Work out the finished part from the listing and answer in its coordinate system (mm). Coordinates: 2 decimals unless noted, no trailing zeros. Loops run counter-clockwise (first coordinate to the right, second up) from the corner with the lowest first, then second, coordinate; pieces in that order, holes last. Notation, with made-up numbers: (56.25, -29.5) -> (80.25, -29.5) arc R25 cw to (80.25, -17.5) -> close; hole circle Ø11 at (73, 47.25). An arc over 180 degrees is marked (long way). Use a Markdown table: item, result.
from build123d import *

# Parameters (mm, degrees)
F0_R     = 12.6233535656
F0_R_2   = 19.05
F1_DEPTH = 3.175


with BuildPart() as f1:
    # F0 (on Front) → F1 (new body)
    with BuildSketch(Plane.XZ):
        with BuildLine():
            ThreePointArc((68.11386007, -24.7914176064), (71.3840419736, -12.586932592), (72.485255884, 0))
            ThreePointArc((72.485255884, 0), (71.3840419736, 12.586932592), (68.11386007, 24.7914176064))
            ThreePointArc((68.11386007, 24.7914176064), (62.7740729954, 36.242627942), (55.526927478, 46.5926243672))
            ThreePointArc((55.526927478, 46.5926243672), (46.5926243672, 55.526927478), (36.242627942, 62.7740729954))
            ThreePointArc((36.242627942, 62.7740729954), (24.7914176064, 68.11386007), (12.586932592, 71.3840419736))
            ThreePointArc((12.586932592, 71.3840419736), (0, 72.485255884), (-12.586932592, 71.3840419736))
            ThreePointArc((-12.586932592, 71.3840419736), (-24.7914176064, 68.11386007), (-36.242627942, 62.7740729954))
            ThreePointArc((-36.242627942, 62.7740729954), (-46.5926243672, 55.526927478), (-55.526927478, 46.5926243672))
            ThreePointArc((-55.526927478, 46.5926243672), (-62.7740729954, 36.242627942), (-68.11386007, 24.7914176064))
            ThreePointArc((-68.11386007, 24.7914176064), (-71.3840419736, 12.586932592), (-72.485255884, 0))
            ThreePointArc((-72.485255884, 0), (-71.3840419736, -12.586932592), (-68.11386007, -24.7914176064))
            ThreePointArc((-68.11386007, -24.7914176064), (-62.7740729954, -36.242627942), (-55.526927478, -46.5926243672))
            ThreePointArc((-55.526927478, -46.5926243672), (-46.5926243672, -55.526927478), (-36.242627942, -62.7740729954))
            ThreePointArc((-36.242627942, -62.7740729954), (-24.7914176064, -68.11386007), (-12.586932592, -71.3840419736))
            ThreePointArc((-12.586932592, -71.3840419736), (0, -72.485255884), (12.586932592, -71.3840419736))
            ThreePointArc((12.586932592, -71.3840419736), (24.7914176064, -68.11386007), (36.242627942, -62.7740729954))
            ThreePointArc((36.242627942, -62.7740729954), (46.5926243672, -55.526927478), (55.526927478, -46.5926243672))
            ThreePointArc((55.526927478, -46.5926243672), (62.7740729954, -36.242627942), (68.11386007, -24.7914176064))
        make_face()
        with Locations((-25.4, -38.1)):
            Circle(F0_R, mode=Mode.SUBTRACT)
        with Locations((25.4, -38.1)):
            Circle(F0_R, mode=Mode.SUBTRACT)
        with Locations((-25.4, 38.1)):
            Circle(F0_R, mode=Mode.SUBTRACT)
        Circle(F0_R_2, mode=Mode.SUBTRACT)
        with Locations((25.4, 38.1)):
            Circle(F0_R, mode=Mode.SUBTRACT)
        with BuildLine():
            Line((87.4346938634, -13.8457773117), (72.485255884, 0))
            ThreePointArc((72.485255884, 0), (71.3840419736, -12.586932592), (68.11386007, -24.7914176064))
            Line((68.11386007, -24.7914176064), (87.4346938634, -13.8457773117))
        make_face()
        with BuildLine():
            ThreePointArc((68.11386007, 24.7914176064), (71.3840419736, 12.586932592), (72.485255884, 0))
            Line((72.485255884, 0), (86.8972713647, 16.893651758))
            Line((86.8972713647, 16.893651758), (68.11386007, 24.7914176064))
        make_face()
        with BuildLine():
            ThreePointArc((55.526927478, 46.5926243672), (62.7740729954, 36.242627942), (68.11386007, 24.7914176064))
            Line((68.11386007, 24.7914176064), (75.8787554723, 45.5954571019))
            Line((75.8787554723, 45.5954571019), (55.526927478, 46.5926243672))
        make_face()
        with BuildLine():
            Line((77.4262018835, -42.9152012956), (68.11386007, -24.7914176064))
            ThreePointArc((68.11386007, -24.7914176064), (62.7740729954, -36.242627942), (55.526927478, -46.5926243672))
            Line((55.526927478, -46.5926243672), (77.4262018835, -42.9152012956))
        make_face()
        with BuildLine():
            ThreePointArc((36.242627942, 62.7740729954), (46.5926243672, 55.526927478), (55.526927478, 46.5926243672))
            Line((55.526927478, 46.5926243672), (55.7081418188, 68.797777402))
            Line((55.7081418188, 68.797777402), (36.242627942, 62.7740729954))
        make_face()
        with BuildLine():
            Line((58.0789672675, -66.8084186424), (55.526927478, -46.5926243672))
            ThreePointArc((55.526927478, -46.5926243672), (46.5926243672, -55.526927478), (36.242627942, -62.7740729954))
            Line((36.242627942, -62.7740729954), (58.0789672675, -66.8084186424))
        make_face()
        with BuildLine():
            ThreePointArc((12.586932592, 71.3840419736), (24.7914176064, 68.11386007), (36.242627942, 62.7740729954))
            Line((36.242627942, 62.7740729954), (28.8183040973, 83.7020704004))
            Line((28.8183040973, 83.7020704004), (12.586932592, 71.3840419736))
        make_face()
        with BuildLine():
            Line((31.7265520446, -82.6435547137), (36.242627942, -62.7740729954))
            ThreePointArc((36.242627942, -62.7740729954), (24.7914176064, -68.11386007), (12.586932592, -71.3840419736))
            Line((12.586932592, -71.3840419736), (31.7265520446, -82.6435547137))
        make_face()
        with BuildLine():
            ThreePointArc((-12.586932592, 71.3840419736), (0, 72.485255884), (12.586932592, 71.3840419736))
            Line((12.586932592, 71.3840419736), (-1.5474464112, 88.5106583975))
            Line((-1.5474464112, 88.5106583975), (-12.586932592, 71.3840419736))
        make_face()
        with BuildLine():
            Line((1.5474464112, -88.5106583975), (12.586932592, -71.3840419736))
            ThreePointArc((12.586932592, -71.3840419736), (0, -72.485255884), (-12.586932592, -71.3840419736))
            Line((-12.586932592, -71.3840419736), (1.5474464112, -88.5106583975))
        make_face()
        with BuildLine():
            ThreePointArc((-36.242627942, 62.7740729954), (-24.7914176064, 68.11386007), (-12.586932592, 71.3840419736))
            Line((-12.586932592, 71.3840419736), (-31.7265520446, 82.6435547137))
            Line((-31.7265520446, 82.6435547137), (-36.242627942, 62.7740729954))
        make_face()
        with BuildLine():
            Line((-28.8183040973, -83.7020704004), (-12.586932592, -71.3840419736))
            ThreePointArc((-12.586932592, -71.3840419736), (-24.7914176064, -68.11386007), (-36.242627942, -62.7740729954))
            Line((-36.242627942, -62.7740729954), (-28.8183040973, -83.7020704004))
        make_face()
        with BuildLine():
            ThreePointArc((-55.526927478, 46.5926243672), (-46.5926243672, 55.526927478), (-36.242627942, 62.7740729954))
            Line((-36.242627942, 62.7740729954), (-58.0789672675, 66.8084186424))
            Line((-58.0789672675, 66.8084186424), (-55.526927478, 46.5926243672))
        make_face()
        with BuildLine():
            Line((-55.7081418188, -68.797777402), (-36.242627942, -62.7740729954))
            ThreePointArc((-36.242627942, -62.7740729954), (-46.5926243672, -55.526927478), (-55.526927478, -46.5926243672))
            Line((-55.526927478, -46.5926243672), (-55.7081418188, -68.797777402))
        make_face()
        with BuildLine():
            ThreePointArc((-68.11386007, 24.7914176064), (-62.7740729954, 36.242627942), (-55.526927478, 46.5926243672))
            Line((-55.526927478, 46.5926243672), (-77.4262018835, 42.9152012956))
            Line((-77.4262018835, 42.9152012956), (-68.11386007, 24.7914176064))
        make_face()
        with BuildLine():
            Line((-75.8787554723, -45.5954571019), (-55.526927478, -46.5926243672))
            ThreePointArc((-55.526927478, -46.5926243672), (-62.7740729954, -36.242627942), (-68.11386007, -24.7914176064))
            Line((-68.11386007, -24.7914176064), (-75.8787554723, -45.5954571019))
        make_face()
        with BuildLine():
            ThreePointArc((-72.485255884, 0), (-71.3840419736, 12.586932592), (-68.11386007, 24.7914176064))
            Line((-68.11386007, 24.7914176064), (-87.4346938634, 13.8457773117))
            Line((-87.4346938634, 13.8457773117), (-72.485255884, 0))
        make_face()
        with BuildLine():
            Line((-86.8972713647, -16.893651758), (-68.11386007, -24.7914176064))
            ThreePointArc((-68.11386007, -24.7914176064), (-71.3840419736, -12.586932592), (-72.485255884, 0))
            Line((-72.485255884, 0), (-86.8972713647, -16.893651758))
        make_face()
    extrude(amount=F1_DEPTH)


solid = f1.part
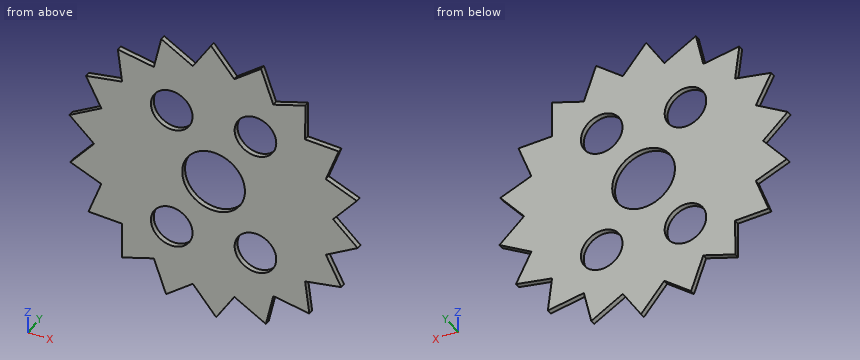
Q1. Section C-C on z = -38.1 is taken. Determine the outline of the cut face in (x, y) (3 decimals), and give its area (3 significant figures).
Solved:
| item | result |
|---|---|
| outline | (-73.081, -3.175) -> (-38.023, -3.175) -> (-38.023, 0) -> (-73.081, 0) -> close; (-12.777, -3.175) -> (12.777, -3.175) -> (12.777, 0) -> (-12.777, 0) -> close; (38.023, -3.175) -> (74.952, -3.175) -> (74.952, 0) -> (38.023, 0) -> close |
| area | 310 mm² |
Q2. Given pin 1 Ø15 at (x, z) = (-25.4, 38.1) entering from -Y; pin 2 Ø10 at (x, z) = (59, -39) entering from +Y; pin 3 Ø1.5 at (x, y) = (16.5, -1) entering from -Z, each flat-ended and moving along its own axis, determine where each tip first touches the part or whether it passes through.
Solved:
| item | result |
|---|---|
| pin 1 | through |
| pin 2 | y = 0 |
| pin 3 | z = -74.13 |
Q3. Section D-D on x = -61 is taken. Determine the outline of the cut face in (y, z) (3 decimals), and give its area (3 significant figures).
Solved:
| item | result |
|---|---|
| outline | (-3.175, -46.324) -> (0, -46.324) -> (0, 45.674) -> (-3.175, 45.674) -> close |
| area | 292 mm² |
Q4. Section A-A on x = 25.4 is taken. Determine the outline of the cut face in (y, z) (3 decimals), and give its area (3 significant figures).
Solved:
| item | result |
|---|---|
| outline | (-3.175, -78.922) -> (0, -78.922) -> (0, -50.723) -> (-3.175, -50.723) -> close; (-3.175, -25.477) -> (0, -25.477) -> (0, 25.477) -> (-3.175, 25.477) -> close; (-3.175, 50.723) -> (0, 50.723) -> (0, 81.108) -> (-3.175, 81.108) -> close |
| area | 348 mm² |
Q5. Consider line 1 (Z direction, x = -25.4, y = -2); line 2 (X direction, y = -1.45, z = 73.5); line 3 (X direction, y = -2.7, z = -35). Determine where each line is inside the solid, lowest interval first. Write a range as [from, to].
Solved:
| item | result |
|---|---|
| line 1 | [-81.11, -50.72], [-25.48, 25.48], [50.72, 78.92] |
| line 2 | [-33.8, -16.18], [-11.22, 10.84], [15.38, 32.44] |
| line 3 | [-71.92, -37.64], [-13.16, 13.16], [37.64, 73.36] |
Q6. Section B-B on y = -0.9 is taken. State how many separate pieces and enclosed holes the cut face has, and give its area (3 significant figures).
Solved:
| item | result |
|---|---|
| separate pieces | 1 |
| enclosed holes | 5 |
| area | 16,900 mm² |
